Part model, mm, in its own coordinate system. A direction names the side the tool comes from. Coordinates: 2 decimals unless noted, no trailing zeros. Write each loop counter-clockwise with the first axis right and the second up, starting at its lowest first coordinate (ties: lowest second). Pieces come first, ordered by that corner, then holes. Notation, with made-up numbers: M 1.5,21.25 L 43.5,21.25 A31 cw 43.5,60.25 Z; hole C 31,14 d10. An arc over 180 degrees is marked long. Use a Markdown table: item, result. Add a question column.
Q1. Slice it at B-B on y = 7. Write the cut outline in (x, z).
Q2. Slice it at A-A on y = 19.5. Write the cut outline in (x, z), then the cut area to 3 significant figures.
Q3. Slice it at C-C on z = 13. Write the cut outline in (x, y).
Q4. Pin check, flat tips, straight feed: pin 1 Ø2.5 at (x, z) = (38.5, -1) entering from -Y; pin 2 Ø12 at (y, z) = (4, 1) entering from -X; pin 3 Ø7.5 at (y, z) = (12, 0.5) entering from +X. Stop position of each tip, or through.
Q5. Mould opens along X. For faces 1 (the flat face through (-1.1, 12, 8.3)), 2 (the flat face through (24, 21, 0)), 3 (the flat face through (3, 5, 6)) say: released by +X, released by -X, zero draft, split by the parting line, or undercut.
Q6. Wall check: L1, parallel to Z at x = -0.5, y = 7; L2, parallel to Y at x = -19, z = -12; L3, parallel to X at y = 21.75, z = 16.5. Give the ranges that are in metal, low to high. Write a range as from..to.
Q7. Slice it at D-D on y = 27.5. Write the cut outline in (x, z), then the cut area to 3 significant figures.
Q8. Tool access for faces 4 (the flat face through (33, 13, 0)), 5 (the flat face through (57, 23, 7.5)), 6 (the cylindrical face through (16, 7, 0)), 7 (the flat face through (47, 15, 4)): list every direction of +Z, -Z, +X, -X, +Y, -Y with a clear straight run to the whole face (end or side of a thin tool).
from build123d import *

# Parameters (mm, degrees)
BOSS_EXTRUDE1_DEPTH = 18
FILLET1_RADIUS      = 18
FILLET1_LENGTH      = 12
CUT_EXTRUDE1_DEPTH  = 36
CUT_EXTRUDE2_DEPTH  = 36


with BuildPart() as part:
    # Sketch1 → Boss-Extrude1 (new, symmetric)
    with BuildSketch(Plane.XY):
        Polygon((-27, 12), (-27, 0), (0, 0), (21, 6.021653101), (33, 6.021653101), (33, 21), (42, 21), (42, 15), (60, 15), (60, 30), (24, 30), (24, 12), align=None)
    extrude(amount=BOSS_EXTRUDE1_DEPTH, both=True)

    # Fillet1: full round fillet: the end face becomes a half cylinder, R = half its width
    fillet1_face = Plane((-27, 6, 0), x_dir=(0, -1, 0), z_dir=(-1, 0, 0))  # on the end face: x along it, z out of the body
    fillet1_slab = fillet1_face.offset(-FILLET1_RADIUS / 2) * Box(FILLET1_LENGTH, 2 * FILLET1_RADIUS, FILLET1_RADIUS, mode=Mode.PRIVATE)  # the body's end, R deep
    fillet1_round = Plane((-9, 6, 0), x_dir=(-1, 0, 0), z_dir=(0, -1, 0)) * Cylinder(FILLET1_RADIUS, FILLET1_LENGTH, mode=Mode.PRIVATE)  # its axis R under the face
    add(fillet1_slab - fillet1_round, mode=Mode.SUBTRACT)

    # Sketch3 → Cut-Extrude1 (cut)
    with BuildSketch(Plane(origin=(0, 12, 0), x_dir=(1, 0, 0), z_dir=(0, 1, 0))):
        with BuildLine():
            Line((10, -6), (-4, -6))
            ThreePointArc((-4, -6), (-10, 0), (-4, 6))
            Line((-4, 6), (10, 6))
            ThreePointArc((10, 6), (16, 0), (10, -6))
        make_face()
    extrude(amount=-CUT_EXTRUDE1_DEPTH, mode=Mode.SUBTRACT)

    # Chamfer1: read off the stored shape, not the designer's step
    # Chamfer1: loft between two sections, ruled curve by curve
    chamfer1_from = [
        Edge.make_three_point_arc((10, 10, 6), (14.242640687, 10, 4.242640687), (16, 10, 0)),
        Edge.make_three_point_arc((16, 10, 0), (14.242640687, 10, -4.242640687), (10, 10, -6)),
        Edge.make_three_point_arc((-4, 10, -6), (-8.242640687, 10, -4.242640687), (-10, 10, 0)),
        Edge.make_three_point_arc((-10, 10, 0), (-8.242640687, 10, 4.242640687), (-4, 10, 6)),
        Edge.make_line((-4, 10, 6), (10, 10, 6)),
        Edge.make_line((10, 10, -6), (-4, 10, -6)),
    ]
    chamfer1_to = [
        Edge.make_three_point_arc((10, 12, 8), (15.656854249, 12, 5.656854249), (18, 12, 0)),
        Edge.make_three_point_arc((18, 12, 0), (15.656854249, 12, -5.656854249), (10, 12, -8)),
        Edge.make_three_point_arc((-4, 12, -8), (-9.656854249, 12, -5.656854249), (-12, 12, 0)),
        Edge.make_three_point_arc((-12, 12, 0), (-9.656854249, 12, 5.656854249), (-4, 12, 8)),
        Edge.make_line((-4, 12, 8), (10, 12, 8)),
        Edge.make_line((10, 12, -8), (-4, 12, -8)),
    ]
    chamfer1 = Solid(Shell([*[Face.make_surface_from_curves(chamfer1_from[k], chamfer1_to[k]) for k in range(6)], Face(Wire(chamfer1_from)), Face(Wire(chamfer1_to))]))
    add(chamfer1, mode=Mode.SUBTRACT)

    # Sketch4 → Cut-Extrude2 (cut)
    with BuildSketch(Plane(origin=(0, 30, 0), x_dir=(1, 0, 0), z_dir=(0, 1, 0))):
        with BuildLine():
            Line((54, 7.5), (65.591333802, 7.5))
            ThreePointArc((65.591333802, 7.5), (73.091333802, 0), (65.591333802, -7.5))
            Line((65.591333802, -7.5), (54, -7.5))
            ThreePointArc((54, -7.5), (46.5, 0), (54, 7.5))
        make_face()
    extrude(amount=-CUT_EXTRUDE2_DEPTH, mode=Mode.SUBTRACT)


solid = part.part
Recorded:
| question | item | result |
|---|---|---|
| 1 | outline | M -9,-18 L 33,-18 L 33,18 L -9,18 A18 ccw Z; hole M -4,-6 L 10,-6 A6 ccw 10,6 L -4,6 A6 ccw Z |
| 2 | outline | M 24,-18 L 33,-18 L 33,18 L 24,18 Z; M 42,-18 L 60,-18 L 60,-7.5 L 54,-7.5 A7.5 cw 54,7.5 L 60,7.5 L 60,18 L 42,18 Z |
| 2 | area | 794 mm² |
| 3 | outline | M -21.45,0 L 0,0 L 21,6.02 L 33,6.02 L 33,21 L 42,21 L 42,15 L 60,15 L 60,30 L 24,30 L 24,12 L -21.45,12 Z |
| 4 | pin 1 | y = 21 |
| 4 | pin 2 | x = -27 |
| 4 | pin 3 | x = 47.02 |
| 5 | face 1 | zero draft |
| 5 | face 2 | released by -X |
| 5 | face 3 | undercut |
| 6 | L1 | -18..-6, 6..18 |
| 6 | L2 | 0..12 |
| 6 | L3 | 24..60 |
| 7 | outline | M 24,-18 L 60,-18 L 60,-7.5 L 54,-7.5 A7.5 cw 54,7.5 L 60,7.5 L 60,18 L 24,18 Z |
| 7 | area | 1,120 mm² |
| 8 | face 4 | +Z, -Z, -Y |
| 8 | face 5 | +X, +Y, -Y |
| 8 | face 6 | +Y, -Y |
| 8 | face 7 | +Z, -Z, +X, -Y |
